Geometry: final body of the model. Coordinates: model frame, mm. Face numbers are marked on the shaded views. A direction names the side the tool comes from. Coordinates: 2 decimals unless noted, no trailing zeros. Order: outer loops, then holes, each group sorted by start corner. A loop starts at its lowest first (then second) coordinate and runs counter-clockwise, first axis right, second up. Notation, with made-up numbers: M -10.75,7 L 13.25,7 A16 ccw 13.25,17 Z; hole C 36,-21.75 d3. An arc over 180 degrees is marked long. Use CSV: the item, a comma, the result in double quotes. Start each with the question number.
Q1. Section query B-B, the plane x = 0. Output: boundary loops of the cut face in (y, z).
Q2. Section query C-C, the plane z = 32. Output: boundary loops of the cut face in (x, y).
Q3. Ray query, probe 1 along X at (y, z) = (-5, 26); probe 2 along Z at (x, y) = (-7.75, -8.25); probe 3 along Z at (x, y) = (3.25, -10). Return the intervals inside material, ascending.
Q4. Section query D-D, the plane y = -7. Output: boundary loops of the cut face in (x, z).
Q5. Mould query, pull axis Z, two halves, no side actions, for the marked faces 1, 2, 3 and 4. Classes: +Z half, -Z half, draft (parallel to the pull), parting line (faces both ways), or undercut.
Q6. Access query for the marked faces 5, 6, 7 and 8. Directions: +Z, -Z, +X, -X, +Y, -Y. A direction counts if a zero-diameter tool reaches every point of the face in a straight line with its end or side. Return the directions, or none.
Q7. First-contact query: P1, Ø5, axis at x = -1.5, z = 6.5, coming from the -Y side; P2, Ø1.3, axis at x = -7.5, z = 2, coming from the +Y side; P3, Ø9.5, axis at x = 0, y = -0.3, coming from the +Z side. Flat tips, straight axial feed; report the tip coordinate or a pass-through.
Q8. Section query A-A, the plane z = 4. Output: boundary loops of the cut face in (x, y), and give its area (3 significant figures).
from build123d import *

# Parameters (mm, degrees)
BOSS_EXTRUDE1_DEPTH      = 8.55
SKETCH2_W                = 10.7
SKETCH2_H                = 10.8
CUT_EXTRUDE1_DEPTH       = 12
SKETCH3_R                = 6
BOSS_EXTRUDE2_DEPTH      = 23
SKETCH4_R                = 4.2
CUT_EXTRUDE2_DEPTH       = 29.152131358
BOSS_EXTRUDE5_DEPTH      = 17.1
CUT_EXTRUDE4_REACH       = 36.056
SKETCH10_W               = 8.1
SKETCH10_H               = 1.5
SKETCH7_R                = 2.2
CUT_EXTRUDE3_DEPTH       = 40.626944786
CUT_EXTRUDE9_START       = -22
CUT_EXTRUDE9_DEPTH       = 22
BOSS_EXTRUDE6_DEPTH      = 1.553
SKETCH16_W               = 28
SKETCH16_H               = 2.5
BOSS_EXTRUDE8_DEPTH      = 7
CUT_EXTRUDE8_DEPTH       = 6.997
CUT_EXTRUDE10_REACH      = 42.722
SKETCH19_R               = 2.83394
CUT_EXTRUDE11_DEPTH      = 41.664727171
CUT_EXTRUDE11_DEPTH_BACK = 41.664727171
SKETCH20_R               = 1.7
SKETCH21_R               = 2.75
CUT_EXTRUDE12_DEPTH      = 41.664727171
CUT_EXTRUDE13_REACH      = 47.107


with BuildPart() as part:
    # Sketch1 → Boss-Extrude1 (new, symmetric)
    with BuildSketch(Plane(origin=(0, 0, 0), x_dir=(0, 0, -1), z_dir=(1, 0, 0))):
        Polygon((0, 0), (0, -8.09401), (-21.6094, -13.8), (-35, -13.8), (-35, 0), align=None)
    extrude(amount=BOSS_EXTRUDE1_DEPTH, both=True)

    # Sketch2 → Cut-Extrude1 (cut)
    with BuildSketch(Plane.XY.offset(35)):
        with Locations((0, -5.4)):
            Rectangle(SKETCH2_W, SKETCH2_H)
    extrude(amount=-CUT_EXTRUDE1_DEPTH, mode=Mode.SUBTRACT)

    # Sketch3 → Boss-Extrude2 (add, through all)
    with BuildSketch(Plane.XY.offset(23)):
        with Locations((0, -0.30175)):
            Circle(SKETCH3_R)
    extrude(amount=-BOSS_EXTRUDE2_DEPTH)

    # Sketch4 → Cut-Extrude2 (cut, through all)
    with BuildSketch(Plane.XY.offset(23)):
        with Locations((0, -0.30175)):
            Circle(SKETCH4_R)
    extrude(amount=-CUT_EXTRUDE2_DEPTH, mode=Mode.SUBTRACT)

    # Sketch8 → Boss-Extrude5 (add, through all)
    with BuildSketch(Plane(origin=(8.55, 0, 0), x_dir=(0, 0, -1), z_dir=(1, 0, 0))):
        Polygon((-29.2, -13.8), (-29.2, -15.3), (-28.2, -15.3), (-26.7, -13.8), align=None)
    extrude(amount=-BOSS_EXTRUDE5_DEPTH)

    # Cut-Extrude4: up to this plane
    cut_extrude4_end = Plane(origin=(-8.55, -15.3, 28.2), z_dir=(0, -0.7071067811865467, -0.7071067811865483))
    # Sketch10 → Cut-Extrude4 (cut, up to the surface)
    with BuildSketch(Plane.XY.offset(29.2), mode=Mode.PRIVATE) as cut_extrude4_sk1:
        with Locations((0, -14.55)):
            Rectangle(SKETCH10_W, SKETCH10_H)
    cut_extrude4_tool1 = split(extrude(cut_extrude4_sk1.sketch, amount=-CUT_EXTRUDE4_REACH, mode=Mode.PRIVATE), bisect_by=cut_extrude4_end, keep=Keep.BOTH, mode=Mode.PRIVATE)
    add(cut_extrude4_tool1.solids().sort_by_distance((0, -14.55, 29.2))[0], mode=Mode.SUBTRACT)

    # Sketch7 → Cut-Extrude3 (cut, through all)
    with BuildSketch(Plane(origin=(0, -10.8, 0), x_dir=(1, 0, 0), z_dir=(0, 1, 0))):
        with Locations(Location((0, -27, 0), (0, 0, 180))):
            Circle(SKETCH7_R)
    extrude(amount=-CUT_EXTRUDE3_DEPTH, mode=Mode.SUBTRACT)

    # Sketch18 → Cut-Extrude9 (cut)
    with BuildSketch(Plane(origin=(0, 0, 0), x_dir=(-1, 0, 0), z_dir=(0, 0, -1)).offset(CUT_EXTRUDE9_START)):
        with BuildLine():
            Line((-5.35, -3.017905371), (-5.35, -13.8))
            Line((-5.35, -13.8), (5.35, -13.8))
            Line((5.35, -13.8), (5.35, -3.017905371))
            ThreePointArc((5.35, -3.017905371), (0, -6.30175), (-5.35, -3.017905371))
        make_face()
    extrude(amount=CUT_EXTRUDE9_DEPTH, mode=Mode.SUBTRACT)

    # Sketch14 → Boss-Extrude6 (add, symmetric)
    with BuildSketch(Plane(origin=(0, 0, 0), x_dir=(0, 0, -1), z_dir=(1, 0, 0))):
        Polygon((-20, -13.8), (-17.001986023, -10.59401), (0, -10.59401), (0, -4.8), (-22, -4.8), (-22, -13.8), align=None)
    extrude(amount=BOSS_EXTRUDE6_DEPTH, both=True)

    # Sketch16 → Boss-Extrude8 (add)
    with BuildSketch(Plane(origin=(0, 0, 0), x_dir=(-1, 0, 0), z_dir=(0, 0, -1))):
        with Locations((-1.44, -9.34401)):
            Rectangle(SKETCH16_W, SKETCH16_H)
    extrude(amount=-BOSS_EXTRUDE8_DEPTH)

    # Sketch17 → Cut-Extrude8 (cut)
    with BuildSketch(Plane(origin=(8.55, 0, 0), x_dir=(0, 0, -1), z_dir=(1, 0, 0))):
        Polygon((-7, -8.09401), (-17.4, -8.09401), (-21.6094, -13.8), (-7, -13.8), align=None)
    extrude(amount=-CUT_EXTRUDE8_DEPTH, mode=Mode.SUBTRACT)

    # Sketch19 → Cut-Extrude10 (cut, up to next)
    with BuildSketch(Plane(origin=(1.553, 0, 0), x_dir=(0, 0, -1), z_dir=(1, 0, 0)), mode=Mode.PRIVATE) as cut_extrude10_sk1:
        with Locations((-9.50021991, -11.92822)):
            Circle(SKETCH19_R)
    cut_extrude10_tool1 = extrude(cut_extrude10_sk1.sketch, amount=-CUT_EXTRUDE10_REACH, mode=Mode.PRIVATE) & part.part
    add(cut_extrude10_tool1.solids().sort_by_distance((1.553, -11.92822, 9.50022))[0], mode=Mode.SUBTRACT)

    # Sketch20 → Cut-Extrude11 (cut, two sides: drawn at the far end of the back side and taken through both)
    with BuildSketch(Plane(origin=(0, -8.09401, 0), x_dir=(1, 0, 0), z_dir=(0, 1, 0)).offset(-CUT_EXTRUDE11_DEPTH_BACK)):
        with Locations(Location((-9.06279, -4.126, 0), (0, 0, 270))):
            Circle(SKETCH20_R)
        with Locations(Location((10.39013, -4.126, 0), (0, 0, 270))):
            Circle(SKETCH20_R)
    extrude(amount=CUT_EXTRUDE11_DEPTH + CUT_EXTRUDE11_DEPTH_BACK, mode=Mode.SUBTRACT)

    # Sketch21 → Cut-Extrude12 (cut, through all)
    with BuildSketch(Plane(origin=(0, -8.09401, 0), x_dir=(1, 0, 0), z_dir=(0, 1, 0))):
        with Locations((-8.56, -4)):
            Circle(SKETCH21_R)
        with Locations((9.44, -4)):
            Circle(SKETCH21_R)
    extrude(amount=CUT_EXTRUDE12_DEPTH, mode=Mode.SUBTRACT)

    # Sketch22 → Cut-Extrude13 (cut, up to next)
    with BuildSketch(Plane.ZY.offset(8.55), mode=Mode.PRIVATE) as cut_extrude13_sk1:
        Polygon((17.4, -8.09401), (7, -8.09401), (7, -9.942369047), (21.6094, -13.8), align=None)
    cut_extrude13_tool1 = extrude(cut_extrude13_sk1.sketch, amount=-CUT_EXTRUDE13_REACH, mode=Mode.PRIVATE) & part.part
    add(cut_extrude13_tool1.solids().sort_by_distance((-8.55, -10.188689, 14.252315))[0], mode=Mode.SUBTRACT)


solid = part.part
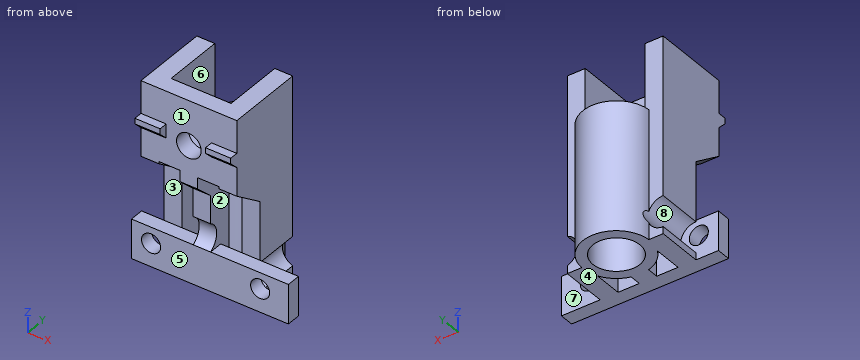
Responses:
1,outline,"M -13.8,20 L -10.59,17 L -10.59,12 A2.83 cw -10.59,7 L -10.59,0 L -4.5,0 L -4.5,23 L -10.8,23 L -10.8,24.8 L -13.8,24.8 Z; M -13.8,29.2 L -10.8,29.2 L -10.8,35 L -13.8,35 Z; M 3.9,0 L 5.7,0 L 5.7,23 L 3.9,23 Z"
2,outline,"M -8.55,-13.8 L 8.55,-13.8 L 8.55,0 L 5.35,0 L 5.35,-10.8 L -5.35,-10.8 L -5.35,0 L -8.55,0 Z"
3,probe 1,"x = -8.55 to -5.35, 5.35 to 8.55"
3,probe 2,"z = 0 to 3.05, 5.21 to 7, 17.52 to 35"
3,probe 3,"z = 0 to 7, 22 to 23"
4,outline,"M -8.55,0 L -5.35,0 L -5.35,22 L -1.55,22 L -1.55,0 L 1.55,0 L 1.55,22 L 5.35,22 L 5.35,0 L 8.55,0 L 8.55,1.4 A2.75 cw 8.55,6.6 L 8.55,35 L 5.35,35 L 5.35,23 L -5.35,23 L -5.35,35 L -8.55,35 L -8.55,6.75 A2.75 cw -8.55,1.25 Z"
5,face 1,"draft"
5,face 2,"undercut"
5,face 3,"undercut"
5,face 4,"-Z half"
6,face 5,"-Z, +X, -X, -Y"
6,face 6,"+Z, +Y"
6,face 7,"+X, +Y"
6,face 8,"-X, +Y"
7,P1,"stops at y = -10.59"
7,P2,"stops at y = 0"
7,P3,"stops at z = 23"
8,outline,"M -12.56,-10.59 L -10.76,-10.59 L -10.76,-8.09 L -12.56,-8.09 Z; M -7.37,-10.59 L 8.69,-10.59 L 8.69,-8.09 L 6.69,-8.09 L 6.69,0 L 5.99,0 A6 ccw -5.81,1.2 L -5.81,-8.09 L -7.37,-8.09 Z; M 12.09,-10.59 L 15.44,-10.59 L 15.44,-8.09 L 12.09,-8.09 Z; hole M -5.35,-8.09 L -1.55,-8.09 L -1.55,-6.1 A6 cw -5.35,-3.02 Z; hole C 0,-0.3 d8.4; hole M 1.55,-8.09 L 5.35,-8.09 L 5.35,-3.02 A6 cw 1.55,-6.1 Z"
8,area,"128 mm²"
